Autodesk Inventor part; units mm, degrees
ref_plane "YZ Plane" through (0, 0, 0) normal (1, 0, 0) x (0, 1, 0)
ref_plane "XZ Plane" through (0, 0, 0) normal (0, 1, 0) x (-1, 0, 0)
ref_plane "XY Plane" through (0, 0, 0) normal (0, 0, 1) x (1, 0, 0)
sketch "Sketch1" plane through (0, 0, 0) normal (0, 0, 1) x (1, 0, 0)
  line L0 (-95.25, -76.2) -> (95.25, -76.2)
  line L1 (95.25, -76.2) -> (95.25, 76.2)
  line L2 (95.25, 76.2) -> (-95.25, 76.2)
  line L3 (-95.25, 76.2) -> (-95.25, -76.2)
  line L4 (-95.25, -76.2) -> (95.25, 76.2) construction
  line L5 (95.25, -76.2) -> (-95.25, 76.2) construction
  point P0 (0, 0)
  dimension "width" = 190.5
  dimension "length" = 152.4
extrude "Extrusion1" add sketch "Sketch1" along normal mid plane 3.175
sketch "Sketch2" plane through (0, 0, 1.5875) normal (0, 0, 1) x (1, 0, 0)
  line L0 (-95.25, -76.2) -> (-95.25, 76.2) construction
  line L1 (-95.25, 76.2) -> (95.25, 76.2) construction
  line L2 (95.25, 76.2) -> (95.25, -76.2) construction
  line L3 (95.25, -76.2) -> (-95.25, -76.2) construction
  point P0 (0, 0)
  point P1 (-82.55, -63.5)
  point P2 (82.55, 63.5)
  dimension "d4" = 12.7
  dimension "d5" = 12.7
  dimension "d19" = 12.7
  dimension "d20" = 12.7
hole "Hole1" at (-82.55, -63.5, 1.5875) direction (0, 0, -1) diameter 5.1054 end through all
pattern_linear "Rectangular Pattern1" count 8 spacing 25.4 along (0, 1, 0) of "Hole1"
pattern_linear "Rectangular Pattern2" count 7 spacing 25.4 along (1, 0, 0) of "Hole1"
hole "Hole2" at (82.55, 63.5, 1.5875) direction (0, 0, -1) diameter 5.1054 end through all
pattern_linear "Rectangular Pattern3" count 7 spacing 25.4 along (-1, 0, 0) of "Hole2"
pattern_linear "Rectangular Pattern4" count 6 spacing 25.4 along (0, -1, 0) of "Hole2"
properties part number "EL2-C-003" material "Aluminum 6061"
Model file for the job. Use its own axes, mm. Coordinates: 2 decimals unless noted, no trailing zeros. Loops run counter-clockwise (first coordinate to the right, second up) from the corner with the lowest first, then second, coordinate; pieces in that order, holes last. Notation, with made-up numbers: M 40.5,64.25 L 46.5,64.25 A17 ccw 46.5,82.25 Z; hole C 21,51 d8. An arc over 180 degrees is marked long. Use CSV: the item, a comma, the result in double quotes. Start each with the question number.
1. Probe probe 1 along Y at (x, z) = (-44, 1.4); probe 2 along Y at (x, z) = (69.85, -0.45). List the from-to ranges inside material, lowest first. Write a range as [from, to].
2. Band-saw the part on C-C, the plane z = 0.3. Give the number of separate pieces and of enclosed holes in the cut face, then the cut area to 3 significant figures.
3. Two-plate mould, pull along Y, no slides. Class faces 1 (the cylindrical face through (-17.5, 65.53, -0.02)), 2 (the cylindrical face through (-80.285, -39.278, -0.022)), 3 (the flat face through (-1, 1, -1.588)): pulls with the +Y half, pulls with the -Y half, needs draft (parallel to the pull), parting line crosses it, or undercut.
4. Band-saw the part on A-A, the plane x = 19.05. List the corners of the cut face in (y, z), then the cut area to 3 significant figures.
5. Band-saw the part on B-B, the plane y = 12.7. List the corners of the cut face in (x, z), then the cut area to 3 significant figures.
6. Flat gauge pin, fed straight in: pin 1 (6 mm diameter, centred on x = 57.15, y = 63.5, fed in from +Z). Where does the tip first touch, or does it go through?
Entries:
1,probe 1,"y = [-76.2, 60.99], [66.01, 76.2]"
1,probe 2,"y = [-76.2, -66.05], [-60.95, 76.2]"
2,separate pieces,"1"
2,enclosed holes,"24"
2,area,"28,500 mm2"
3,face 1,"undercut"
3,face 2,"undercut"
3,face 3,"needs draft"
4,outline,"M -76.2,-1.59 L -66.05,-1.59 L -66.05,1.59 L -76.2,1.59 Z; M -60.95,-1.59 L 76.2,-1.59 L 76.2,1.59 L -60.95,1.59 Z"
4,area,"468 mm2"
5,outline,"M -95.25,-1.59 L -85.1,-1.59 L -85.1,1.59 L -95.25,1.59 Z; M -80,-1.59 L 80,-1.59 L 80,1.59 L -80,1.59 Z; M 85.1,-1.59 L 95.25,-1.59 L 95.25,1.59 L 85.1,1.59 Z"
5,area,"572 mm2"
6,pin 1,"stops at z = 1.59"
